```python
from build123d import *

# Parameters (mm, degrees)
SKETCH1_W                 = 64
SKETCH1_H                 = 23
BOSS_EXTRUDE1_DEPTH       = 3
F_3_0_3_DIAMETER_HOLE1_D  = 3
FILLET1_R                 = 3
SKETCH5_R                 = 11.5
BOSS_EXTRUDE2_DEPTH       = 3
F_3_0_3_DIAMETER_HOLE2_D  = 3
M3X0_5_TAPPED_HOLE1_D     = 2.5
M3X0_5_TAPPED_HOLE1_DEPTH = 4.748924226
M3X0_5_TAPPED_HOLE1_TIP   = 0.751075774


with BuildPart() as part:
    # Sketch1 → Boss-Extrude1 (new body)
    with BuildSketch(Plane(origin=(0, 0, 0), x_dir=(1, 0, 0), z_dir=(0, 1, 0))):
        Rectangle(SKETCH1_W, SKETCH1_H)
    extrude(amount=-BOSS_EXTRUDE1_DEPTH)

    # Ø3.0 (3) Diameter Hole1 (through all)
    with Locations(Plane(origin=(0, 0, 0), x_dir=(1, 0, 0), z_dir=(0, 1, 0))):
        with Locations((-29, 0), (-29, 9), (-14.5, 9), (-14.5, -9), (-29, -9)):
            f_3_0_3_diameter_hole1 = Hole(F_3_0_3_DIAMETER_HOLE1_D / 2)

    # Mirror1: Ø3.0 (3) Diameter Hole1 across plane
    add(f_3_0_3_diameter_hole1.mirror(Plane(origin=(0, 0, 0), x_dir=(0, 0, 1), z_dir=(1, 0, 0))), mode=Mode.SUBTRACT)

    # Fillet1
    fillet1_edges = [part.edges().sort_by_distance(p)[0] for p in [
        (32, -1.5, 11.5),
        (-32, -1.5, 11.5),
        (-32, -1.5, -11.5),
        (32, -1.5, -11.5),
    ]]
    fillet(fillet1_edges, radius=FILLET1_R)

    # Sketch5 → Boss-Extrude2 (add)
    with BuildSketch(Plane(origin=(0, 0, 0), x_dir=(1, 0, 0), z_dir=(0, 1, 0))):
        with Locations(Location((0, 0, 0), (0, 0, 270))):
            Circle(SKETCH5_R)
    extrude(amount=BOSS_EXTRUDE2_DEPTH)

    # Ø3.0 (3) Diameter Hole2 (through all)
    with Locations(Plane(origin=(0, 3, 0), x_dir=(1, 0, 0), z_dir=(0, 1, 0))):
        with Locations((0, 9), (0, -9)):
            Hole(F_3_0_3_DIAMETER_HOLE2_D / 2)

    # M3x0.5 Tapped Hole1
    with Locations(Plane(origin=(0, 3, 0), x_dir=(1, 0, 0), z_dir=(0, 1, 0))):
        with Locations((-9, 0), (9, 0)):
            Hole(M3X0_5_TAPPED_HOLE1_D / 2, depth=M3X0_5_TAPPED_HOLE1_DEPTH)
            with Locations((0, 0, -(M3X0_5_TAPPED_HOLE1_DEPTH + M3X0_5_TAPPED_HOLE1_TIP / 2))):  # 118° drill point
                Cone(0, M3X0_5_TAPPED_HOLE1_D / 2, M3X0_5_TAPPED_HOLE1_TIP, mode=Mode.SUBTRACT)


solid = part.part
```
Read the model definition and answer for the solid it produces. Units are mm, in the model's axes. A direction names the side the tool comes from. Coordinates: 2 decimals unless noted, no trailing zeros. Order: outer loops, then holes, each group sorted by start corner. A loop starts at its lowest first (then second) coordinate and runs counter-clockwise, first axis right, second up. Notation, with made-up numbers: (66, 62) - (81, 62) arc R25 cw to (81, 100) - close; hole circle Ø4 at (-13.75, 80). An arc over 180 degrees is marked (long way). Answer as a JSON object with one key per item and string values. Group by question number.
Item 1: The mould has two halves that part along Z. Classify faces 1 (the face through (31.1, -1.52, 10.64)), 2 (the face through (-31.14, -1.52, -10.6)), 3 (the face through (9.7, 1.48, 6.18)), 4 (the face through (0.325, -0.042, 10.464)): +Z half, -Z half, draft (parallel to the pull), parting line (faces both ways), or undercut.
Item 2: Section A-A (x = 14.5) is taken. Give the vertices of the cut face in (y, z).
Item 3: Section C-C (z = 2.25) is taken. Give the vertices of the cut face in (x, y).
Item 4: Consider probe 1 along Z at (x, y) = (-14.5, -1); probe 2 along Z at (x, y) = (-29, -0.65); probe 3 along X at (y, z) = (-1.9, -8). Determine where each line is inside the solid, lowest interval first. Write a range as from..to.
Item 5: Flat-ended cylindrical pins translate along their axes: P1, Ø5, axis at x = 14.5, z = 9, coming from the -Y side; P2, Ø5, axis at x = 29, z = 0, coming from the +Y side; P3, Ø2.5, axis at x = 29, z = -9, coming from the -Y side; P4, Ø1.5, axis at x = 2, y = 2, coming from the +Z side. Find the tip coordinate at first contact, or state that the pin passes through.
Item 6: Section B-B (y = 1.75) is taken. Give the vertices of the cut face in (x, z).
Item 7: A tool of negligible diameter and unlimited length cuts with its end or side. For faces 5 (the face through (27.8, -1.5, 0.9)), 6 (the face through (-7.75, 0.59, -0.05)), from which of +Z, -Z, +X, -X, +Y, -Y can it reach the whole face along a straight path? Write none if from no direction.
Item 8: Section D-D (x = 24) is taken. Give the vertices of the cut face in (y, z), plus the area to 3 significant figures.
Results are:
{
 "1": {"face 1": "+Z half", "face 2": "-Z half", "face 3": "parting line", "face 4": "undercut"},
 "2": {"outline": "(-3, -11.5) - (0, -11.5) - (0, -10.5) - (-3, -10.5) - close; (-3, -7.5) - (0, -7.5) - (0, 7.5) - (-3, 7.5) - close; (-3, 10.5) - (0, 10.5) - (0, 11.5) - (-3, 11.5) - close"},
 "3": {"outline": "(-32, -3) - (32, -3) - (32, 0) - (11.28, 0) - (11.28, 3) - (-11.28, 3) - (-11.28, 0) - (-32, 0) - close"},
 "4": {"probe 1": "z = -11.5..-10.5, -7.5..7.5, 10.5..11.5", "probe 2": "z = -11.5..-10.5, -7.5..-1.5, 1.5..7.5, 10.5..11.5", "probe 3": "x = -32..-30.12, -27.88..-15.62, -13.38..-1.12, 1.12..13.38, 15.62..27.88, 30.12..32"},
 "5": {"P1": "stops at y = -3", "P2": "stops at y = 0", "P3": "passes through", "P4": "stops at z = 11.43"},
 "6": {"outline": "circle Ø23 at (0, 0); hole circle Ø2.5 at (-9, 0); hole circle Ø3 at (0, -9); hole circle Ø3 at (0, 9); hole circle Ø2.5 at (9, 0)"},
 "7": {"face 5": "+Y, -Y", "face 6": "+Y"},
 "8": {"outline": "(-3, -11.5) - (0, -11.5) - (0, 11.5) - (-3, 11.5) - close", "area": "69.0 mm^2"}
}
